Print and shaded views of the part. All mm, measured from the part's lowest x, y and z. Round coordinates to 2 decimals unless told otherwise and drop trailing zeros. Loops run counter-clockwise (first coordinate to the right, second up) from the corner with the lowest first, then second, coordinate; pieces in that order, holes last. Notation, with made-up numbers: (32, -34) -> (53, -34) arc R33 cw to (53, -2) -> close; hole circle Ø10 at (55, 48). An arc over 180 degrees is marked (long way). Answer as CSV lines item,"result".
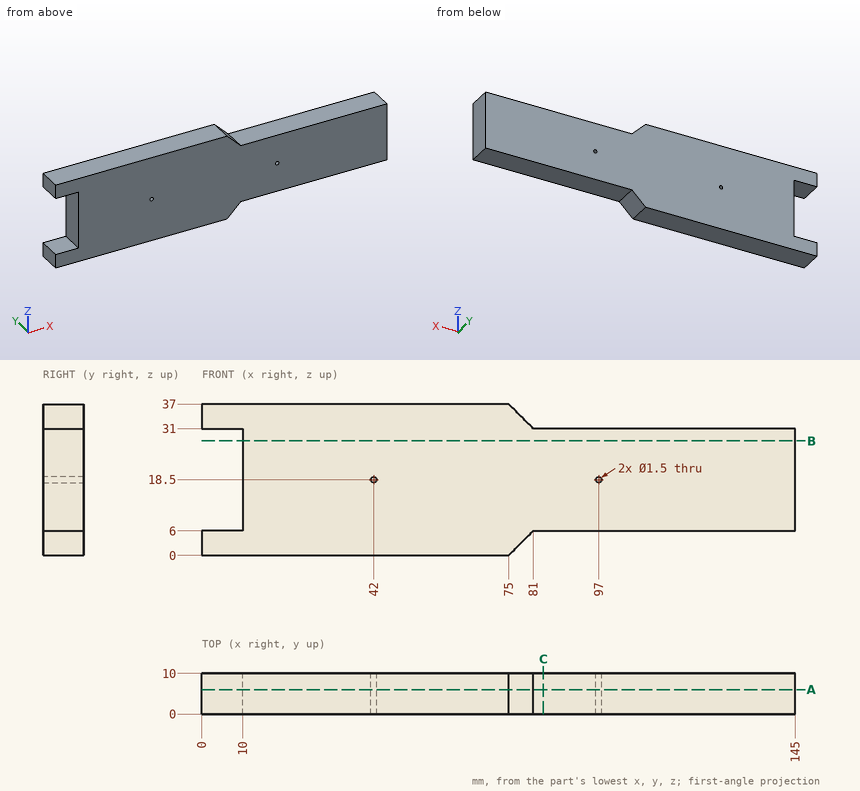
Q1. Drop a flat-ended pin along its axis: pin 1 Ø5 at (x, y) = (100, 3) entering from -Z. Give the stop position or say it passes through.
Results:
pin 1,"z = 6"
Q2. Slice it at A-A, the plane y = 6. Give the cut face in (x, z).
Results:
outline,"(0, 0) -> (75, 0) -> (81, 6) -> (145, 6) -> (145, 31) -> (81, 31) -> (75, 37) -> (0, 37) -> (0, 31) -> (10, 31) -> (10, 6) -> (0, 6) -> close; hole circle Ø1.5 at (42, 18.5); hole circle Ø1.5 at (97, 18.5)"
Q3. Slice it at B-B, the plane z = 28. Give the cut face in (x, y), and give its area (3 significant figures).
Results:
outline,"(10, 0) -> (145, 0) -> (145, 10) -> (10, 10) -> close"
area,"1,350 mm2"
Q4. Slice it at C-C, the plane x = 83.5. Give the cut face in (y, z), and give its area (3 significant figures).
Results:
outline,"(0, 6) -> (10, 6) -> (10, 31) -> (0, 31) -> close"
area,"250 mm2"
Q5. Probe L1, parallel to X at y = 5.5, z = 18.5; L2, parallel to Z at x = 97, y = 5.75; L3, parallel to Z at x = 42, y = 6.25. List the from-to ranges inside material, lowest first. Write a range as [from, to].
Results:
L1,"[10, 41.25], [42.75, 96.25], [97.75, 145]"
L2,"[6, 17.75], [19.25, 31]"
L3,"[0, 17.75], [19.25, 37]"
